```python
from build123d import *

# Parameters (mm, degrees)
SKETCH1_W                      = 82
SKETCH1_H                      = 98
BOSS_EXTRUDE1_DEPTH            = 3
F_3_0_3_DIAMETER_HOLE1_D       = 3
F_3_0_3_DIAMETER_HOLE1_DEPTH   = 30
SKETCH5_W                      = 25
SKETCH5_H                      = 13
CUT_EXTRUDE1_DEPTH             = 10
F_2_3_2_3_DIAMETER_HOLE1_D     = 2.3
F_2_3_2_3_DIAMETER_HOLE1_DEPTH = 30
SKETCH8_R                      = 1.5
CUT_EXTRUDE2_DEPTH             = 10
F_3_0_3_DIAMETER_HOLE2_D       = 3
F_3_0_3_DIAMETER_HOLE2_DEPTH   = 6.5


with BuildPart() as part:
    # Sketch1 → Boss-Extrude1 (new body)
    with BuildSketch(Plane(origin=(0, 0, 0), x_dir=(1, 0, 0), z_dir=(0, 1, 0))):
        Rectangle(SKETCH1_W, SKETCH1_H)
    extrude(amount=BOSS_EXTRUDE1_DEPTH)

    # Ø3.0 (3) Diameter Hole1
    with Locations(Plane(origin=(0, 0, 0), x_dir=(-1, 0, 0), z_dir=(0, -1, 0))):
        with Locations((23, -45.5), (-23, -45.5), (-23, 45.5), (23, 45.5)):
            Hole(F_3_0_3_DIAMETER_HOLE1_D / 2, depth=F_3_0_3_DIAMETER_HOLE1_DEPTH)

    # Sketch5 → Cut-Extrude1 (cut)
    with BuildSketch(Plane.XZ):
        with Locations((-25.5, 0)):
            Rectangle(SKETCH5_W, SKETCH5_H)
        with Locations((25.5, 0)):
            Rectangle(SKETCH5_W, SKETCH5_H)
    extrude(amount=-CUT_EXTRUDE1_DEPTH, mode=Mode.SUBTRACT)

    # Ø2.3 (2.3) Diameter Hole1
    with Locations(Plane(origin=(0, 3, 0), x_dir=(1, 0, 0), z_dir=(0, 1, 0))):
        with Locations((-22.24500144, -31.590736692), (22.24500144, -31.590736692), (22.203117232, 32.633806534), (-22.203117232, 32.633806534)):
            Hole(F_2_3_2_3_DIAMETER_HOLE1_D / 2, depth=F_2_3_2_3_DIAMETER_HOLE1_DEPTH)

    # Sketch8 → Cut-Extrude2 (cut)
    with BuildSketch(Plane.XZ):
        with Locations(Location((5.7, 0.8, 0), (0, 0, 270))):
            Circle(SKETCH8_R)
    extrude(amount=-CUT_EXTRUDE2_DEPTH, mode=Mode.SUBTRACT)

    # Ø3.0 (3) Diameter Hole2
    with Locations(Plane(origin=(0, 0, 0), x_dir=(-1, 0, 0), z_dir=(0, -1, 0))):
        with Locations((-1.4, -5.5), (-8.2, -5.5)):
            Hole(F_3_0_3_DIAMETER_HOLE2_D / 2, depth=F_3_0_3_DIAMETER_HOLE2_DEPTH)


solid = part.part
```
The model under review builds one solid part; all positions refer to its coordinate system, in mm. A direction names the side the tool comes from. Round coordinates to 2 decimals unless told otherwise and drop trailing zeros. Loops run counter-clockwise (first coordinate to the right, second up) from the corner with the lowest first, then second, coordinate; pieces in that order, holes last. Notation, with made-up numbers: M 40,-3.75 L 91,-3.75 A18 cw 91,6.25 Z; hole C -39.75,56.25 d3. An arc over 180 degrees is marked long. Put each result on its own line as item: value.
Q1. Consider section A-A, the plane z = -4. Give the boundary of the cut face in (x, y).
Result set:
outline: M -41,0 L -38,0 L -38,3 L -41,3 Z; M -13,0 L 13,0 L 13,3 L -13,3 Z; M 38,0 L 41,0 L 41,3 L 38,3 Z
Q2. Consider section D-D, the plane x = 18.5. Give the boundary of the cut face in (y, z), then the cut area to 3 significant figures.
Result set:
outline: M 0,-49 L 3,-49 L 3,-6.5 L 0,-6.5 Z; M 0,6.5 L 3,6.5 L 3,49 L 0,49 Z
area: 255 mm²
Q3. Machinability: for faces 1 (the flat face through (-1, 1, 49)), 2 (the flat face through (-26, 1, 6.5)), which of the approach directions +Z, -Z, +X, -X, +Y, -Y give a long, thin tool a straight path to every point of the face, cutting with its end or side? Answer none if there is none.
Result set:
face 1: +Z, +X, -X, +Y, -Y
face 2: +Y, -Y
Q4. Consider section B-B, the plane x = 1.4. Give the boundary of the cut face in (y, z).
Result set:
outline: M 0,-49 L 3,-49 L 3,4 L 0,4 Z; M 0,7 L 3,7 L 3,49 L 0,49 Z
Q5. For pin 1 (2 mm diameter, centred on x = 22.5, z = 24.5, fed in from -Y), flat-tipped, find the tip position at first contact; note if it passes through.
Result set:
pin 1: stops at y = 0
Q6. To check wall thickness, follow L1, parallel to X at y = 1.5, z = -4; L2, parallel to X at y = 0.3, z = 31.5; L3, parallel to Z at x = -29.5, y = 0.7. State the ranges of each line that lie inside material, in increasing order.
Result set:
L1: x = -41 to -38, -13 to 13, 38 to 41
L2: x = -41 to -23.39, -21.1 to 21.1, 23.39 to 41
L3: z = -49 to -6.5, 6.5 to 49
Q7. Consider section C-C, the plane y = 1.5. Count the separate pieces of the cut face and the enclosed holes in it, then the cut area to 3 significant figures.
Result set:
separate pieces: 1
enclosed holes: 13
area: 7,320 mm²
Q8. Mouldability with a two-part tool opening along X and no side actions: class faces 3 (the flat face through (41, 1, 1)), 4 (the flat face through (-41, 1, 1)), 5 (the flat face through (-1, 1, -49)), 6 (the cylindrical face through (-23, 2, -44)) as released by +X, released by -X, zero draft, split by the parting line, or undercut.
Result set:
face 3: released by +X
face 4: released by -X
face 5: zero draft
face 6: undercut
